```python
from build123d import *

# Parameters (mm, degrees)
SKETCH1_W             = 40
SKETCH1_H             = 63
BOSS_EXTRUDE1_DEPTH   = 20
SKETCH2_W             = 7.5
SKETCH2_H             = 20
CUT_EXTRUDE1_DEPTH    = 3.2
M8_TAPPED_HOLE1_D     = 6.8
M8_TAPPED_HOLE1_DEPTH = 19.75
M8_TAPPED_HOLE1_TIP   = 2.042926105
M6_TAPPED_HOLE1_D     = 5
M6_TAPPED_HOLE1_DEPTH = 15
M6_TAPPED_HOLE1_TIP   = 1.502151548
CHAMFER1_SIZE         = 1


with BuildPart() as part:
    # Sketch1 → Boss-Extrude1 (new body)
    with BuildSketch(Plane.XY):
        Rectangle(SKETCH1_W, SKETCH1_H)
    extrude(amount=BOSS_EXTRUDE1_DEPTH)

    # Sketch2 → Cut-Extrude1 (cut)
    with BuildSketch(Plane(origin=(0, 31.5, 0), x_dir=(1, 0, 0), z_dir=(0, 1, 0))):
        with Locations((0, -10)):
            Rectangle(SKETCH2_W, SKETCH2_H)
    extrude(amount=-CUT_EXTRUDE1_DEPTH, mode=Mode.SUBTRACT)

    # M8 Tapped Hole1
    with Locations(Plane(origin=(0, -31.5, 0), x_dir=(-1, 0, 0), z_dir=(0, -1, 0))):
        with Locations((-12, -10), (12, -10)):
            Hole(M8_TAPPED_HOLE1_D / 2, depth=M8_TAPPED_HOLE1_DEPTH)
            with Locations((0, 0, -(M8_TAPPED_HOLE1_DEPTH + M8_TAPPED_HOLE1_TIP / 2))):  # 118° drill point
                Cone(0, M8_TAPPED_HOLE1_D / 2, M8_TAPPED_HOLE1_TIP, mode=Mode.SUBTRACT)

    # M6 Tapped Hole1
    with Locations(Plane(origin=(0, 31.5, 0), x_dir=(1, 0, 0), z_dir=(0, 1, 0))):
        with Locations((-14, -10), (14, -10)):
            Hole(M6_TAPPED_HOLE1_D / 2, depth=M6_TAPPED_HOLE1_DEPTH)
            with Locations((0, 0, -(M6_TAPPED_HOLE1_DEPTH + M6_TAPPED_HOLE1_TIP / 2))):  # 118° drill point
                Cone(0, M6_TAPPED_HOLE1_D / 2, M6_TAPPED_HOLE1_TIP, mode=Mode.SUBTRACT)

    # Chamfer1
    chamfer1_edges = [part.edges().sort_by_distance(p)[0] for p in [
        (-20, 0, 20),
        (-11.875, 31.5, 0),
        (0, -31.5, 20),
        (-11.875, 31.5, 20),
        (20, 0, 20),
        (0, -31.5, 0),
        (-20, 0, 0),
        (11.875, 31.5, 0),
        (20, 0, 0),
        (20, -31.5, 10),
        (-20, -31.5, 10),
        (-20, 31.5, 10),
        (20, 31.5, 10),
        (11.875, 31.5, 20),
    ]]
    chamfer(chamfer1_edges, length=CHAMFER1_SIZE)


solid = part.part
```
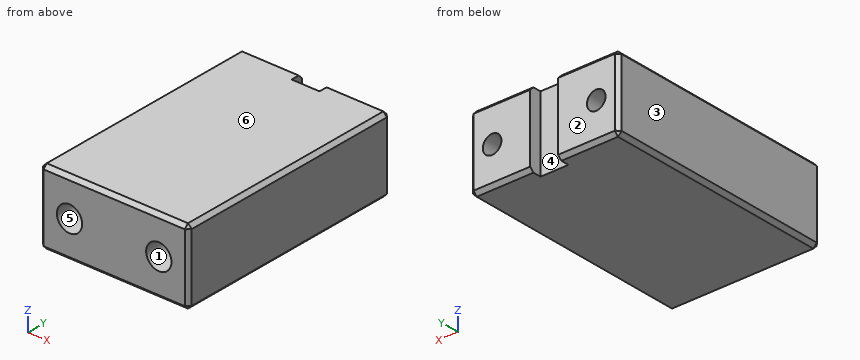
Geometry check sheet. Reference: the model listing, model coordinates, mm. Face numbers are marked on the shaded views. A direction names the side the tool comes from. Coordinates: 2 decimals unless noted, no trailing zeros. Order: outer loops, then holes, each group sorted by start corner. A loop starts at its lowest first (then second) coordinate and runs counter-clockwise, first axis right, second up. Notation, with made-up numbers: M 29,21 L 57,21 A30 ccw 57,55 Z; hole C 61,83 d8. An arc over 180 degrees is marked long. One line per question, with ' | ' between items. Start each with the question number.
Item 1: Gauge pin test, flat ends, axial feed: pin 1 (4.5 mm diameter, centred on x = 14, z = 10, fed in from +Y); pin 2 (4 mm diameter, centred on x = -14, z = 10, fed in from +Y); pin 3 (2 mm diameter, centred on x = -0.5, z = 9.5, fed in from +Y). Record the tip position at first contact, or that the pin passes through.
Item 2: Material ranges on L1, parallel to Z at x = 12, y = -26.5; L2, parallel to X at y = 24.5, z = 9; L3, parallel to Z at x = -14, y = 26, recorded low to high. Write a range as [from, to].
Item 3: Cross-section at B-B on y = -22. Enter the section's corners in (x, z).
Item 4: Cross-section at A-A on y = 20. Enter the section's corners in (x, z), then the cut area to 3 significant figures.
Item 5: Set-up check for the marked faces 1 and 2: record each of +Z, -Z, +X, -X, +Y, -Y from which the full face is reachable in a straight line by a thin tool's end or side.
Item 6: Draft check along X on the marked faces 3, 4, 5 and 6. Enter one of: pulls with the +X half, pulls with the -X half, needs draft (parallel to the pull), parting line crosses it, or undercut.
Findings:
1) pin 1: stops at y = 16.35 | pin 2: stops at y = 16.2 | pin 3: stops at y = 28.3
2) L1: z = [0, 6.6], [13.4, 20] | L2: x = [-20, -16.29], [-11.71, 11.71], [16.29, 20] | L3: z = [0, 7.5], [12.5, 20]
3) outline: M -20,1 L -19,0 L 19,0 L 20,1 L 20,19 L 19,20 L -19,20 L -20,19 Z; hole C -12,10 d6.8; hole C 12,10 d6.8
4) outline: M -20,1 L -19,0 L 19,0 L 20,1 L 20,19 L 19,20 L -19,20 L -20,19 Z; hole C -14,10 d5; hole C 14,10 d5 | area: 759 mm²
5) face 1: -Y | face 2: +Z, -Z, +X, -X, +Y
6) face 3: pulls with the -X half | face 4: undercut | face 5: undercut | face 6: needs draft
